from build123d import *

# Parameters (mm, degrees)
ESQUISSE1_R        = 23.5
BOSS_EXTRU_1_DEPTH = 10
CHANFREIN1_SIZE    = 25.8965397
CHANFREIN1_SIZE_2  = 30


with BuildPart() as part:
    # Esquisse1 → Boss.-Extru.1 (new body)
    with BuildSketch(Plane.XY):
        with BuildLine():
            Line((85, 226.846291066), (56.715728753, 198.562019819))
            Line((56.715728753, 198.562019819), (34.130206535, 198.562019819))
            Line((34.130206535, 198.562019819), (47.084901509, 272.031745907))
            ThreePointArc((47.084901509, 272.031745907), (85, 303.846291066), (122.915098491, 272.031745907))
            Line((122.915098491, 272.031745907), (135.869793465, 198.562019819))
            Line((135.869793465, 198.562019819), (113.284271247, 198.562019819))
            Line((113.284271247, 198.562019819), (85, 226.846291066))
        make_face()
        with Locations((85, 265.346291066)):
            Circle(ESQUISSE1_R, mode=Mode.SUBTRACT)
    extrude(amount=BOSS_EXTRU_1_DEPTH)

    # Chanfrein1
    # the kernel refuses this chamfer: 30, 25.8965397 mm, written as the material it takes off along each edge
    with BuildSketch(Plane(origin=(34.130206535, 198.562019819, -77.150489639), x_dir=(0.9993171132668053, -0.036950062680586405, 0), z_dir=(0, 0, 1)), Plane(origin=(135.869793465, 198.562019819, -77.150489639), x_dir=(-0.13714088742803301, 0.9905515519120909, 0), z_dir=(0, 0, 1))) as chanfrein1_piece_1:
        Polygon((CHANFREIN1_SIZE * 0.999317113282, CHANFREIN1_SIZE * 0.0369500626812), (CHANFREIN1_SIZE_2 * 0.137140887428, CHANFREIN1_SIZE_2 * 0.990551551912), (0, 0), align=None)
    extrude(amount=164.300979278, mode=Mode.SUBTRACT)


solid = part.part
Source: CAD feature listing. Evaluate the final solid. Frame: model axes, mm. A direction names the side the tool comes from. Give positions to 0.01 mm unless a question says otherwise; leave off trailing zeros. Order: outer loops, then holes, each group sorted by start corner. A loop starts at its lowest first (then second) coordinate and runs counter-clockwise, first axis right, second up. Notation, with made-up numbers: (86.25, -35.5) -> (128.25, -35.5) arc R30 cw to (128.25, -2.5) -> close; hole circle Ø7 at (56.25, 33). An arc over 180 degrees is marked (long way). Write item = value, one per line.
Item 1: Contact query for flat-ended pins moving along their axis: pin 1 (1.5 mm diameter, centred on x = 121, z = 3, fed in from +Y); pin 2 (1.5 mm diameter, centred on y = 264, z = 1.5, fed in from -X); pin 3 (3 mm diameter, centred on y = 242.5, z = 4.5, fed in from +X). Output: stop coordinate, or through.
Check result:
pin_1 = 280.83
pin_2 = 45.54
pin_3 = 128.39
Item 2: Mould query, pull axis X, two halves, no side actions, for faces 3 (the face through (120.63, 213.32, 4.93)), 4 (the face through (81.941, 288.646, 4.93)), 5 (the face through (84.25, 303.84, 4.93)). Classes: +X half, -X half, draft (parallel to the pull), parting line (faces both ways), or undercut.
Check result:
face_3 = +X half
face_4 = undercut
face_5 = parting line
Item 3: Ray query, probe 1 along Y at (x, z) = (85, 8.25); probe 2 along Y at (x, z) = (98.5, 6.5); probe 3 along X at (y, z) = (260, 1). Return the intervals inside material, ascending.
Check result:
probe_1 = 226.85 to 241.85, 288.85 to 303.85
probe_2 = 213.35 to 246.11, 284.58 to 301.4
probe_3 = 44.96 to 62.12, 107.88 to 125.04
Item 4: Section query D-D (y = 239). Output: boundary loops of the cut face in (x, z), then the cut area to 3 significant figures.
Check result:
outline = (41.26, 0) -> (128.74, 0) -> (128.74, 10) -> (41.26, 10) -> close
area = 875 mm²
Item 5: Section query C-C (z = 2.5). Output: boundary loops of the cut face in (x, y), then the cut area to 3 significant figures.
Check result:
outline = (39.34, 228.11) -> (58.66, 200.51) -> (85, 226.85) -> (109.58, 202.27) -> (131.37, 224.07) -> (122.92, 272.03) arc R38.5 ccw to (47.08, 272.03) -> close; hole circle Ø47 at (85, 265.35)
area = 5,060 mm²
Item 6: Section query B-B (x = 66). Output: boundary loops of the cut face in (y, z).
Check result:
outline = (207.85, 0) -> (251.52, 0) -> (251.52, 10) -> (207.85, 10) -> close; (279.18, 0) -> (298.83, 0) -> (298.83, 10) -> (279.18, 10) -> close
Item 7: Section query A-A (y = 210.5). Output: boundary loops of the cut face in (x, z).
Check result:
outline = (51.67, 0) -> (68.65, 0) -> (68.65, 10) -> (51.67, 10) -> close; (101.35, 0) -> (117.81, 0) -> (117.81, 10) -> (101.35, 10) -> close
Item 8: Set-up query: faces 1 (the face through (72.016, 213.862, 4.93)), 2 (the face through (43.158, 249.762, 4.93)). Return all of +Z, -Z, +X, -X, +Y, -Y with unobstructed straight access to the full face (end or side cutting, diameter ignored); none if empty.
Check result:
face_1 = +Z, -Z, -Y
face_2 = +Z, -Z, -X, +Y
